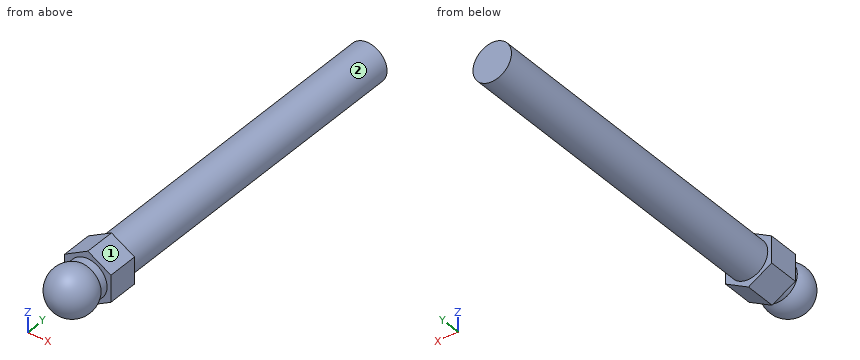
from build123d import *

# Parameters (mm, degrees)
BOSS_EXTRUDE3_DEPTH = 8


with BuildPart() as part:
    # Sketch1 → Revolve1 (revolve)
    with BuildSketch(Plane.XY):
        with BuildLine():
            Line((-5, 3.31662479), (-5, 100))
            Line((-5, 100), (0, 100))
            Line((0, 100), (0, -6))
            ThreePointArc((0, -6), (-5.286764074, -2.837274331), (-5, 3.31662479))
        make_face()
    revolve(axis=Axis((0, 109.494581108, 0), (0, -1, 0)))

    # Sketch4 → Boss-Extrude3 (add)
    with BuildSketch(Plane(origin=(0, 5.31662479, 0), x_dir=(1, 0, 0), z_dir=(0, 1, 0))):
        Polygon((0, 6.92820323), (-6, 3.464101615), (-6, -3.464101615), (0, -6.92820323), (6, -3.464101615), (6, 3.464101615), align=None)
    extrude(amount=BOSS_EXTRUDE3_DEPTH)


solid = part.part
CAD build for the part. Positions are in the model's coordinates, mm. Face numbers are marked on the shaded views. A direction names the side the tool comes from. Coordinates: 2 decimals unless noted, no trailing zeros. Order: outer loops, then holes, each group sorted by start corner. A loop starts at its lowest first (then second) coordinate and runs counter-clockwise, first axis right, second up.
Item 1: Band-saw the part on A-A on z = 0. List the corners of the cut face in (x, y).
Check sheet entries:
outline: (-6, 5.32) - (-5, 5.32) - (-5, 3.32) arc R6 ccw (long way) to (5, 3.32) - (5, 5.32) - (6, 5.32) - (6, 13.32) - (5, 13.32) - (5, 100) - (-5, 100) - (-5, 13.32) - (-6, 13.32) - close
Item 2: 3-axis set-ups, long thin cutter, end or side, ignore diameter. For the marked faces 1 and 2: which of +Z, -Z, +X, -X, +Y, -Y reach the whole face in a straight line?
Check sheet entries:
face 1: +Z, +X, +Y, -Y
face 2: +Y
Item 3: Drill centre lines: L1, parallel to Y at x = -4.75, z = 1.25; L2, parallel to Y at x = 0, z = -0.5; L3, parallel to X at y = 88, z = 0. Where is each one in solid material? Low to high.
Check sheet entries:
L1: y = -3.45 to 100
L2: y = -5.98 to 100
L3: x = -5 to 5
Item 4: Pin check, flat tips, straight feed: pin 1 Ø3.5 at (x, z) = (-1.5, -1.5) entering from -Y; pin 2 Ø3 at (y, z) = (30, 2) entering from +X; pin 3 Ø6 at (x, y) = (-3.5, 27.5) entering from -Z. Stop position of each tip, or through.
Check sheet entries:
pin 1: stops at y = -5.99
pin 2: stops at x = 4.97
pin 3: stops at z = -4.97
Item 5: Band-saw the part on C-C on y = 55. List the corners of the cut face in (x, z), plus the area to 3 significant figures.
Check sheet entries:
outline: circle Ø10 at (0, 0)
area: 78.5 mm2
Item 6: Band-saw the part on B-B on x = 2.5. List the corners of the cut face in (y, z).
Check sheet entries:
outline: (3.32, -4.33) - (5.32, -4.33) - (5.32, -5.48) - (13.32, -5.48) - (13.32, -4.33) - (100, -4.33) - (100, 4.33) - (13.32, 4.33) - (13.32, 5.48) - (5.32, 5.48) - (5.32, 4.33) - (3.32, 4.33) arc R5.45 ccw (long way) to start
